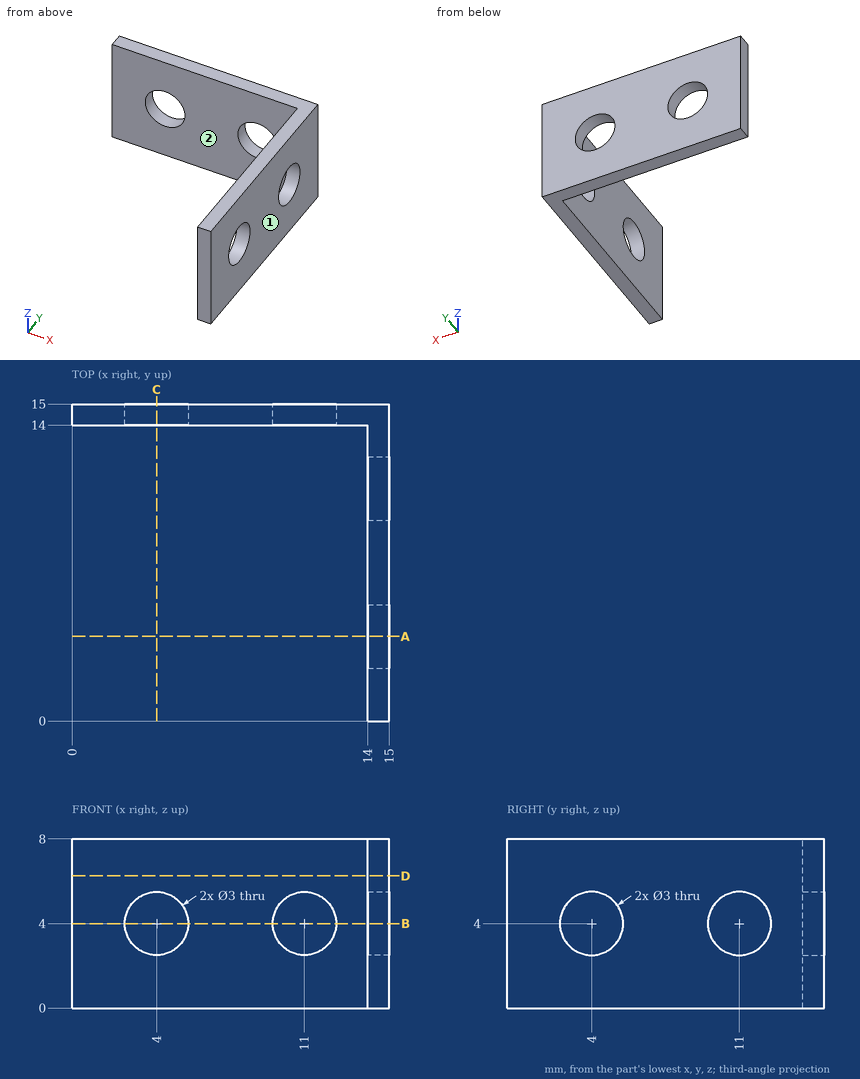
Source: three-view drawing plus pictorial views. Frame: mm from the lowest corner of the part. A direction names the side the tool comes from. Give positions to 0.01 mm unless a question says otherwise; leave off trailing zeros. Write each loop counter-clockwise with the first axis right and the second up, starting at its lowest first coordinate (ties: lowest second). Pieces come first, ordered by that corner, then holes.
(1) Cut plane D-D, the plane z = 6.25. Return loops of the section in (x, y).
(2) Cut plane A-A, the plane y = 4. Return loops of the section in (x, z), then the cut area to 3 significant figures.
(3) Cut plane B-B, the plane z = 4. Return loops of the section in (x, y).
(4) Ray query, line 1 (X direction, y = 14.4, z = 4); line 2 (X direction, y = 14.75, z = 4.75). Return the intervals inside material, ascending.
(5) Access query for the marked faces 1 and 2. Directions: +Z, -Z, +X, -X, +Y, -Y. A direction counts if a zero-diameter tool reaches every point of the face in a straight line with its end or side. Return the directions, or none.
(6) First-contact query: P1, Ø1, axis at x = 2, y = 13, coming from the -Z side; P2, Ø1.5, axis at x = 7.5, z = 2.5, coming from the -Y side; P3, Ø4, axis at y = 11, z = 4, coming from the -X side. Flat tips, straight axial feed; report the tip coordinate or a pass-through.
Values follow:
1. outline: (0, 14) - (14, 14) - (14, 0) - (15, 0) - (15, 15) - (0, 15) - close
2. outline: (14, 0) - (15, 0) - (15, 2.5) - (14, 2.5) - close; (14, 5.5) - (15, 5.5) - (15, 8) - (14, 8) - close
2. area: 5.00 mm2
3. outline: (0, 14) - (2.5, 14) - (2.5, 15) - (0, 15) - close; (5.5, 14) - (9.5, 14) - (9.5, 15) - (5.5, 15) - close; (12.5, 14) - (14, 14) - (14, 12.5) - (15, 12.5) - (15, 15) - (12.5, 15) - close; (14, 0) - (15, 0) - (15, 2.5) - (14, 2.5) - close; (14, 5.5) - (15, 5.5) - (15, 9.5) - (14, 9.5) - close
4. line 1: x = 0 to 2.5, 5.5 to 9.5, 12.5 to 15
4. line 2: x = 0 to 2.7, 5.3 to 9.7, 12.3 to 15
5. face 1: +Z, -Z, +X, +Y, -Y
5. face 2: +Z, -Z, -X, -Y
6. P1: passes through
6. P2: stops at y = 14
6. P3: stops at x = 14
